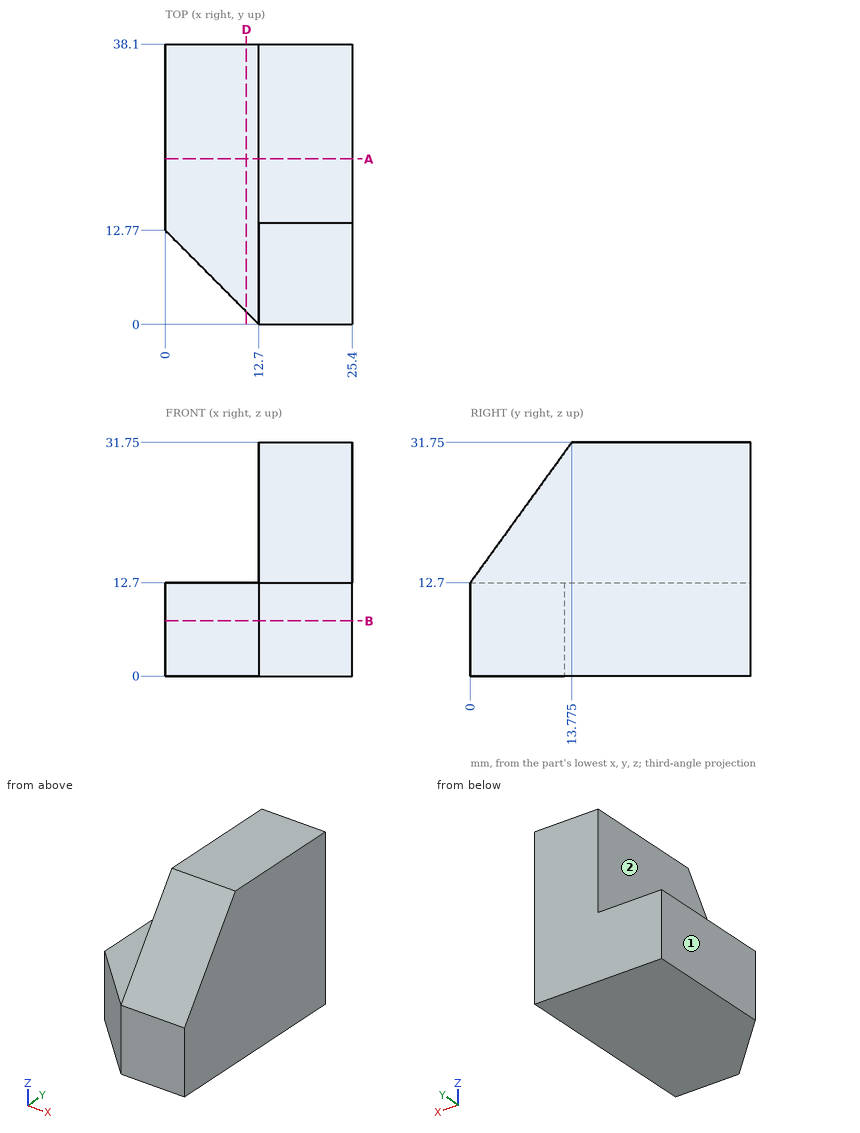
Can you work these out from the drawing? Everything is in mm from the part's minimum corner. A direction names the side the tool comes from. Give positions to 0.01 mm unless a question says otherwise; leave off trailing zeros. Loops run counter-clockwise (first coordinate to the right, second up) from the corner with the lowest first, then second, coordinate; pieces in that order, holes last. Notation, with made-up numbers: M -39.5,52 L -16.5,52 A21 cw -16.5,62 Z; hole C -23.5,-22.75 d8. An arc over 180 degrees is marked long. Use CSV: the item, a comma, the result in double quotes. Start each with the question number.
1. If I drill on L1, parallel to X at y = 29, z = 21.5; L2, parallel to Z at x = 5.5, y = 17.5; L3, parallel to X at y = 12, z = 6.5 (1 decimal), over which ranges is the centre line in solid material (lowest first)?
2. Imagine slicing it at D-D, the plane x = 11. Write out the boundary of the cut face in (y, z).
3. Imagine slicing it at A-A, the plane y = 22.5. Write out the boundary of the cut face in (x, z).
4. On a 3-axis mill with a long thin cutter (end or side, diameter ignored), from which of +Z, -Z, +X, -X, +Y, -Y can I reach the whole of each face in a straight line? I mean the marked faces 1 and 2. Say none if no direction works.
5. For P1, Ø5.5, axis at y = 25.5, z = 21.5, coming from the -X side; P2, Ø4, axis at x = 9, y = 16.5, coming from the +Z side, each with a flat end and sliding along its axis, tell me the tip position at first contact or that it passes through.
6. Imagine slicing it at B-B, the plane z = 7.5. Write out the boundary of the cut face in (x, y).
Response values:
1,L1,"12.7 to 25.4"
1,L2,"0 to 12.7"
1,L3,"0.8 to 25.4"
2,outline,"M 1.71,0 L 38.1,0 L 38.1,12.7 L 1.71,12.7 Z"
3,outline,"M 0,0 L 25.4,0 L 25.4,31.75 L 12.7,31.75 L 12.7,12.7 L 0,12.7 Z"
4,face 1,"+Z, -Z, -X, +Y, -Y"
4,face 2,"+Z, -X, +Y, -Y"
5,P1,"x = 12.7"
5,P2,"z = 12.7"
6,outline,"M 0,12.77 L 12.7,0 L 25.4,0 L 25.4,38.1 L 0,38.1 Z"
